from build123d import *

# Parameters (mm, degrees)
BOSS_EXTRU_1_DEPTH      = 23.5
ESQUISSE2_W             = 20.710678119
ESQUISSE2_H             = 1.4
ESQUISSE2_W_2           = 1.4
ESQUISSE2_H_2           = 20.710678119
ENL_V_MAT_EXTRU_1_DEPTH = 15
ESQUISSE3_R             = 35
ENL_V_MAT_EXTRU_2_DEPTH = 20.5
CHANFREIN1_SIZE         = 4
CONG_1_R                = 3


with BuildPart() as part:
    # Esquisse1 → Boss.-Extru.1 (new body)
    with BuildSketch(Plane(origin=(0, 0, 0), x_dir=(1, 0, 0), z_dir=(0, 1, 0))):
        with BuildLine():
            Line((41.821047333, -5), (63.639610307, -5))
            ThreePointArc((63.639610307, -5), (68.639610307, 0), (63.639610307, 5))
            Line((63.639610307, 5), (41.821047333, 5))
            ThreePointArc((41.821047333, 5), (38.723786728, 6.074827807), (36.958134852, 8.837209302))
            ThreePointArc((36.958134852, 8.837209302), (26.870057685, 26.870057685), (8.837209302, 36.958134852))
            ThreePointArc((8.837209302, 36.958134852), (6.074827807, 38.723786728), (5, 41.821047333))
            Line((5, 41.821047333), (5, 63.639610307))
            ThreePointArc((5, 63.639610307), (0, 68.639610307), (-5, 63.639610307))
            Line((-5, 63.639610307), (-5, 41.821047333))
            ThreePointArc((-5, 41.821047333), (-6.074827807, 38.723786728), (-8.837209302, 36.958134852))
            ThreePointArc((-8.837209302, 36.958134852), (-26.870057685, 26.870057685), (-36.958134852, 8.837209302))
            ThreePointArc((-36.958134852, 8.837209302), (-38.723786728, 6.074827807), (-41.821047333, 5))
            Line((-41.821047333, 5), (-63.639610307, 5))
            ThreePointArc((-63.639610307, 5), (-68.639610307, 0), (-63.639610307, -5))
            Line((-63.639610307, -5), (-41.821047333, -5))
            ThreePointArc((-41.821047333, -5), (-38.723786728, -6.074827807), (-36.958134852, -8.837209302))
            ThreePointArc((-36.958134852, -8.837209302), (-30.152523014, -23.126291443), (-18.11627907, -33.403599097))
            ThreePointArc((-18.11627907, -33.403599097), (15.480011603, -34.704023409), (36.958134852, -8.837209302))
            ThreePointArc((36.958134852, -8.837209302), (38.723786728, -6.074827807), (41.821047333, -5))
        make_face()
    extrude(amount=-BOSS_EXTRU_1_DEPTH)

    # Esquisse2 → Enlèv. mat.-Extru.1 (cut)
    with BuildSketch(Plane.XZ.offset(23.5)):
        with Locations((55.35533906, 0)):
            Rectangle(ESQUISSE2_W, ESQUISSE2_H)
        with Locations((0, -55.35533906)):
            Rectangle(ESQUISSE2_W_2, ESQUISSE2_H_2)
        with Locations((-55.35533906, 0)):
            Rectangle(ESQUISSE2_W, ESQUISSE2_H)
    extrude(amount=-ENL_V_MAT_EXTRU_1_DEPTH, mode=Mode.SUBTRACT)

    # Esquisse3 → Enlèv. mat.-Extru.2 (cut)
    with BuildSketch(Plane.XZ.offset(23.5)):
        with Locations(Location((0, 0, 0), (0, 0, 270))):
            Circle(ESQUISSE3_R)
    extrude(amount=-ENL_V_MAT_EXTRU_2_DEPTH, mode=Mode.SUBTRACT)

    # Chanfrein1
    chanfrein1_edges = [part.edges().sort_by_distance(p)[0] for p in [
        (0, -3, 35),
    ]]
    chamfer(chanfrein1_edges, length=CHANFREIN1_SIZE)

    # Congé1
    cong_1_edges = [part.edges().sort_by_distance(p)[0] for p in [
        (68.639610307, 0, 0),
        (52.73032882, 0, -5),
        (38.723786728, 0, -6.074827807),
        (26.870057685, 0, -26.870057685),
        (6.074827807, 0, -38.723786728),
        (5, 0, -52.73032882),
        (0, 0, -68.639610307),
        (-5, 0, -52.73032882),
        (-6.074827807, 0, -38.723786728),
        (-26.870057685, 0, -26.870057685),
        (-38.723786728, 0, -6.074827807),
        (-52.73032882, 0, -5),
        (-68.639610307, 0, 0),
        (-52.73032882, 0, 5),
        (-38.723786728, 0, 6.074827807),
        (0, 0, 38),
        (38.723786728, 0, 6.074827807),
        (52.73032882, 0, 5),
    ]]
    fillet(cong_1_edges, radius=CONG_1_R)


solid = part.part
Source: CAD feature listing. Evaluate the final solid. Frame: model axes, mm. A direction names the side the tool comes from. Coordinates: 2 decimals unless noted, no trailing zeros. Order: outer loops, then holes, each group sorted by start corner. A loop starts at its lowest first (then second) coordinate and runs counter-clockwise, first axis right, second up. Notation, with made-up numbers: M -37,75.5 L -29,75.5 A32 cw -29,107.5 Z; hole C 68,63 d4. An arc over 180 degrees is marked long. Write each question's results on one line, items separated by ' | '. Start each with the question number.
1. Section C-C, the plane y = -5.5. Return the cut outline in (x, z).
2. Section A-A, the plane y = -12.25. State how many separate pieces and enclosed holes the cut face has, then the cut area to 3 significant figures.
3. Material intervals for L1, parallel to X at y = -12, z = 0; L2, parallel to X at y = -20.25, z = -57, sorted ascending.
4. Section B-B, the plane x = -53.5. Return the cut outline in (y, z), then the cut area to 3 significant figures.
5. Reachability of faces 4 (the face through (-0.7, -16, -56)), 5 (the face through (4.14, -0.9, -52.88)), 6 (the face through (53, -13, 5)), 7 (the face through (53, -13, -5)) from +Z, -Z, +X, -X, +Y, -Y: full face, straight path, thin tool, end or side. Return the list, or none.
6. Draft query along X for faces 1 (the face through (5, -13, -53)), 2 (the face through (52.58, -0.9, -4.14)), 3 (the face through (-21, -15, 28)). Return one class per face: +X half, -X half, draft (parallel to the pull), parting line (faces both ways), or undercut.
7. Pin query (flat end, axial travel): pin 1 (1.5 mm diameter, centred on x = 26.5, y = -18.5, fed in from -Z); pin 2 (0.7 mm diameter, centred on y = -12.5, z = 0.5, fed in from -X); pin 3 (12 mm diameter, centred on x = 54, y = -14.5, fed in from -Z); pin 4 (1.1 mm diameter, centred on x = -58.5, z = -0.5, fed in from -Y). Return the tip coordinate at first contact, or that it passes through.
Solution:
1) outline: M -63.64,-5 L -41.82,-5 A5 cw -36.96,-8.84 A38 ccw -8.84,-36.96 A5 cw -5,-41.82 L -5,-63.64 A5 ccw 5,-63.64 L 5,-41.82 A5 cw 8.84,-36.96 A38 ccw 36.96,-8.84 A5 cw 41.82,-5 L 63.64,-5 A5 ccw 63.64,5 L 41.82,5 A5 cw 36.96,8.84 A38 ccw -36.96,8.84 A5 cw -41.82,5 L -63.64,5 A5 ccw Z; hole C 0,0 d67
2) separate pieces: 1 | enclosed holes: 4 | area: 1,510 mm²
3) L1: -68.64 to -65.71, -45 to -35, 35 to 45, 65.71 to 68.64 | L2: -5 to -0.7, 0.7 to 5
4) outline: M -23.5,-5 L -3,-5 A3 ccw 0,-2 L 0,2 A3 ccw -3,5 L -23.5,5 L -23.5,0.7 L -8.5,0.7 L -8.5,-0.7 L -23.5,-0.7 Z | area: 210 mm²
5) face 4: -Y | face 5: -Z, +X, +Y | face 6: +Z, +X, +Y, -Y | face 7: -Z, +X, +Y, -Y
6) face 1: +X half | face 2: draft | face 3: undercut
7) pin 1: z = -27.95 | pin 2: x = -68.64 | pin 3: z = -5 | pin 4: y = -23.5
